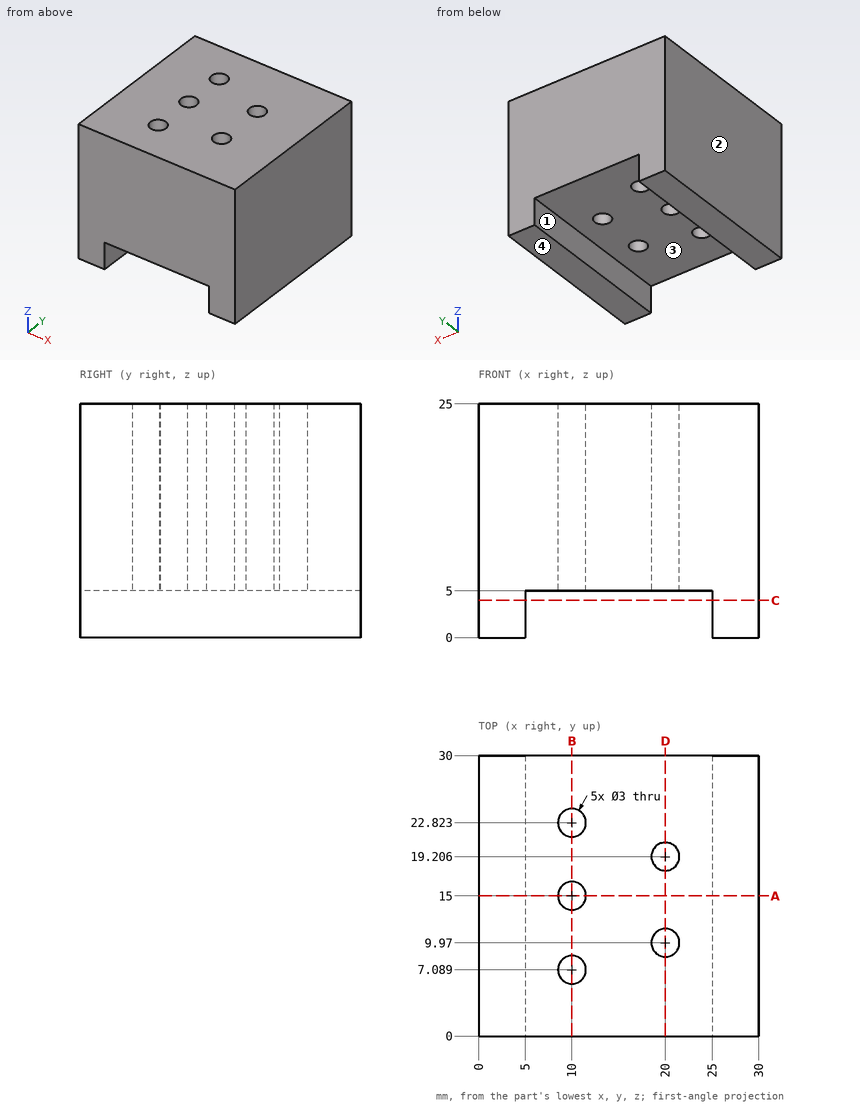
Answer from the drawing. Dimensions are ordinates in mm from the lowest x, y and z of the part. Give positions to 0.01 mm unless a question says otherwise; leave off trailing zeros. Loops run counter-clockwise (first coordinate to the right, second up) from the corner with the lowest first, then second, coordinate; pieces in that order, holes last. Notation, with made-up numbers: (32, 49.5) - (71, 49.5) arc R24 cw to (71, 65.5) - close; hole circle Ø9 at (81.25, -38.5). An arc over 180 degrees is marked (long way). Answer as CSV lines item,"result". Start each with the question number.
Item 1: A cutting plane is placed at D-D on x = 20. Determine the outline of the cut face in (y, z) (1 decimal), then the cut area to 3 significant figures.
Item 2: A cutting plane is placed at B-B on x = 10. Determine the outline of the cut face in (y, z).
Item 3: Find the intervals of material crossed by line 1 (Y direction, x = 10, z = 13.5); line 2 (Y direction, x = 20, z = 20.5) (1 decimal); line 3 (Y direction, x = 11, z = 5.25) (1 decimal), in increasing order. Write a range as from..to.
Item 4: Each of these flat-tipped pins is pushed along its axis until it touches: pin 1 (6 mm diameter, centred on x = 20, y = 17, fed in from -Z); pin 2 (2.5 mm diameter, centred on x = 20, y = 9.97, fed in from +Z). Where does it stop, or does it pass through?
Item 5: A cutting plane is placed at C-C on z = 4. Determine the outline of the cut face in (x, y).
Item 6: The mould has two halves that part along X. Classify the marked faces 1, 2, 3 and 4: +X half, -X half, draft (parallel to the pull), parting line (faces both ways), or undercut.
Item 7: A cutting plane is placed at A-A on y = 15. Determine the outline of the cut face in (x, z), then the cut area to 3 significant figures.
Found:
1,outline,"(0, 5) - (8.5, 5) - (8.5, 25) - (0, 25) - close; (11.5, 5) - (17.7, 5) - (17.7, 25) - (11.5, 25) - close; (20.7, 5) - (30, 5) - (30, 25) - (20.7, 25) - close"
1,area,"480 mm^2"
2,outline,"(0, 5) - (5.59, 5) - (5.59, 25) - (0, 25) - close; (8.59, 5) - (13.5, 5) - (13.5, 25) - (8.59, 25) - close; (16.5, 5) - (21.32, 5) - (21.32, 25) - (16.5, 25) - close; (24.32, 5) - (30, 5) - (30, 25) - (24.32, 25) - close"
3,line 1,"y = 0..5.59, 8.59..13.5, 16.5..21.32, 24.32..30"
3,line 2,"y = 0..8.5, 11.5..17.7, 20.7..30"
3,line 3,"y = 0..6, 8.2..13.9, 16.1..21.7, 23.9..30"
4,pin 1,"stops at z = 5"
4,pin 2,"passes through"
5,outline,"(0, 0) - (5, 0) - (5, 30) - (0, 30) - close; (25, 0) - (30, 0) - (30, 30) - (25, 30) - close"
6,face 1,"undercut"
6,face 2,"-X half"
6,face 3,"undercut"
6,face 4,"draft"
7,outline,"(0, 0) - (5, 0) - (5, 5) - (8.5, 5) - (8.5, 25) - (0, 25) - close; (11.5, 5) - (25, 5) - (25, 0) - (30, 0) - (30, 25) - (11.5, 25) - close"
7,area,"590 mm^2"
